Verification items for the finished model (mm, model axes). Face numbers are marked on the shaded views. A direction names the side the tool comes from. Give positions to 0.01 mm unless a question says otherwise; leave off trailing zeros. Write each loop counter-clockwise with the first axis right and the second up, starting at its lowest first coordinate (ties: lowest second). Pieces come first, ordered by that corner, then holes. Notation, with made-up numbers: (71, 27.25) -> (88, 27.25) arc R23 cw to (88, 46.25) -> close; hole circle Ø6 at (-34.75, -9.75). An arc over 180 degrees is marked (long way). Write item = value, one per line.
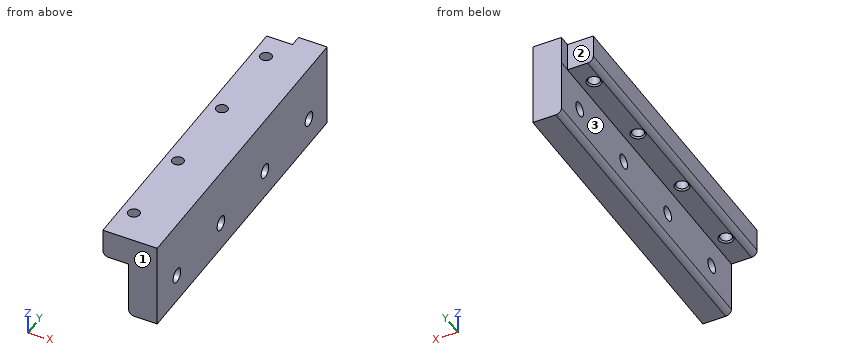
Autodesk Inventor part; units mm, degrees
ref_plane "YZ Plane" through (0, 0, 0) normal (1, 0, 0) x (0, 1, 0)
ref_plane "XZ Plane" through (0, 0, 0) normal (0, 1, 0) x (-1, 0, 0)
ref_plane "XY Plane" through (0, 0, 0) normal (0, 0, 1) x (1, 0, 0)
sketch "Skizze2" plane through (0, 0, 0) normal (0, 1, 0) x (-1, 0, 0)
  line L0 (0, 0) -> (19, 0)
  line L1 (19, 0) -> (19, -10)
  line L2 (19, -10) -> (10, -10)
  line L3 (10, -10) -> (10, -30)
  line L4 (10, -30) -> (0, -30)
  line L5 (0, -30) -> (0, 0)
  dimension "d6" = 10
  dimension "d7" = 20
  dimension "d8" = 10
  dimension "d9" = 9
extrude "Extrusion1" add sketch "Skizze2" along normal blind 112
sketch "Skizze3" plane through (-10, 0, -10) normal (0, 0, -1) x (-1, 0, 0)
  line L0 (0, 112) -> (9, 112)
  point P0 (-10, 0)
  point P1 (4.5, 99)
  point P2 (4.5, 70)
  point P3 (4.5, 41)
  point P4 (4.5, 12)
  point P5 (4.5, 112)
  point P6 (4.5, 112)
  dimension "d12" = 13
  dimension "d13" = 29
  dimension "d14" = 29
  dimension "d15" = 29
hole "Bohrung1" at (-14.5, 99, -10) at (-14.5, 70, -10) at (-14.5, 41, -10) at (-14.5, 12, -10) direction (0, 0, 1) diameter 4 depth 10 countersink diameter 5 countersink angle 90
sketch "Skizze4" plane through (-10, 0, -30) normal (-1, 0, 0) x (0, 0, 1)
  line L0 (0, 112) -> (20, 112)
  line L1 (0, 0) -> (20, 0)
  point P0 (30, 0)
  point P1 (10, 100)
  point P2 (10, 71)
  point P3 (10, 42)
  point P4 (10, 13)
  point P5 (10, 0)
  dimension "d30" = 12
  dimension "d31" = 29
  dimension "d32" = 29
  dimension "d33" = 29
hole "Bohrung2" at (-10, 100, -20) at (-10, 71, -20) at (-10, 42, -20) at (-10, 13, -20) direction (1, 0, 0) diameter 5 end through all
sketch "Skizze5" plane through (-10, 0, -10) normal (0, 0, -1) x (-1, 0, 0)
  line L0 (9, 112) -> (-0.0001, 112)
  line L1 (9, 112) -> (9, 108)
  line L2 (9, 0) -> (9, 112)
  line L3 (9, 108) -> (0, 108)
  line L4 (0, 0) -> (0, 112)
  line L5 (0, 112) -> (0, 108)
  point P0 (-10, 0)
  dimension "d40" = 4
extrude "Extrusion2" cut sketch "Skizze5" against normal up to surface (10 mm away)
fillet "Rundung1" radius 2 2 edges at (-10, 56, -30) (-19, 54, -10)
properties part number "1014_right"
Item 1: Sectioned sample at A-A on z = -5.75. Record the cut outline in (x, y).
Response values:
outline = (-19, 0) -> (0, 0) -> (0, 112) -> (-10, 112) -> (-10, 108) -> (-19, 108) -> close; hole circle Ø4 at (-14.5, 12); hole circle Ø4 at (-14.5, 41); hole circle Ø4 at (-14.5, 70); hole circle Ø4 at (-14.5, 99)
Item 2: Sectioned sample at C-C on y = 61. Record the cut outline in (x, z), then the cut area to 3 significant figures.
Response values:
outline = (-19, -8) arc R2 ccw to (-17, -10) -> (-10, -10) -> (-10, -28) arc R2 ccw to (-8, -30) -> (0, -30) -> (0, 0) -> (-19, 0) -> close
area = 388 mm^2
Item 3: Sectioned sample at B-B on x = -1.5. Record the cut outline in (y, z).
Response values:
outline = (0, -30) -> (112, -30) -> (112, 0) -> (0, 0) -> close; hole circle Ø5 at (13, -20); hole circle Ø5 at (42, -20); hole circle Ø5 at (71, -20); hole circle Ø5 at (100, -20)
Item 4: Set-up check for the marked faces 1, 2 and 3: record each of +Z, -Z, +X, -X, +Y, -Y from which the full face is reachable in a straight line by a thin tool's end or side.
Response values:
face_1 = +Z, -Z, +X, -X, -Y
face_2 = +Z, -Z, -X, +Y
face_3 = -Z, -X, +Y, -Y
Item 5: Go/stop test with flat-tipped pins: P1, Ø9, axis at y = 69, z = -23, coming from the -X side; P2, Ø3.5, axis at x = -14.5, y = 70, coming from the +Z side; P3, Ø5.5, axis at x = -14, y = 38, coming from the -Z side. Record where each tip stops, or that it passes through.
Response values:
P1 = -10
P2 = through
P3 = -10
Item 6: Sectioned sample at D-D on z = -21.25. Record the cut outline in (x, y).
Response values:
outline = (-10, 0) -> (0, 0) -> (0, 10.83) -> (-10, 10.83) -> close; (-10, 15.17) -> (0, 15.17) -> (0, 39.83) -> (-10, 39.83) -> close; (-10, 44.17) -> (0, 44.17) -> (0, 68.83) -> (-10, 68.83) -> close; (-10, 73.17) -> (0, 73.17) -> (0, 97.83) -> (-10, 97.83) -> close; (-10, 102.17) -> (0, 102.17) -> (0, 112) -> (-10, 112) -> close
Item 7: Material ranges on line 1 (Y direction, x = -14.5, z = -3.75); line 2 (Y direction, x = -7.75, z = -20); line 3 (X direction, y = 12, z = -6.75), recorded low to high.
Response values:
line_1 = 0 to 10, 14 to 39, 43 to 68, 72 to 97, 101 to 108
line_2 = 0 to 10.5, 15.5 to 39.5, 44.5 to 68.5, 73.5 to 97.5, 102.5 to 112
line_3 = -19 to -16.5, -12.5 to 0
